Source: CAD feature listing. Evaluate the final solid. Frame: model axes, mm. Coordinates: 2 decimals unless noted, no trailing zeros. Loops run counter-clockwise (first coordinate to the right, second up) from the corner with the lowest first, then second, coordinate; pieces in that order, holes last. Notation, with made-up numbers: (52.5, 27.5) - (62.5, 27.5) arc R14 cw to (62.5, 40.5) - close; hole circle Ø6 at (64, 11.5). An arc over 180 degrees is marked (long way). Use one line per item in the form item = value. Start each with the question number.
Solid Edge part; units mm, degrees
sketch "Sketch1" plane through (0, 0, 0) normal (0, 0, 1) x (1, 0, 0)
  arc A0 (0, 6.3) -> (0.3, 6) centre (0.3, 6.3) ccw
  line L0 (0.3, 6) -> (7.7, 6)
  arc A1 (7.7, 6) -> (8, 6.3) centre (7.7, 6.3) ccw
  line L1 (8, 6.3) -> (8, 8.4)
  arc A2 (8, 8.4) -> (7.9, 8.5) centre (7.9, 8.4) ccw
  line L2 (7.9, 8.5) -> (5.8491, 8.5)
  arc A3 (5.8491, 8.5) -> (2.1509, 8.5) centre (4, 10) cw
  line L3 (2.1509, 8.5) -> (0.1, 8.5)
  arc A4 (0.1, 8.5) -> (0, 8.4) centre (0.1, 8.4) ccw
  line L4 (0, 8.4) -> (0, 6.3)
revolve "RevolvedProtrusion1" add sketch "Sketch1" angle 360 about axis through (100, 0, 0) along (-1, 0, 0)
properties part number "SKF_6001_ir"
(1) Mould query, pull axis Z, two halves, no side actions, for faces 1 (the face through (1.11, -1.84, 8.3)), 2 (the face through (8, 3, -6)), 3 (the face through (4, -6, 0)). Classes: +Z half, -Z half, draft (parallel to the pull), parting line (faces both ways), or undercut.
(2) Contact query for flat-ended pins moving along their axis: pin 1 (1 mm diameter, centred on x = 2.5, y = -6.5, fed in from +Z); pin 2 (2 mm diameter, centred on x = 1, y = -3.5, fed in from -Z); pin 3 (2 mm diameter, centred on x = 6, z = 5.5, fed in from +Y). Output: stop coordinate, or through.
(3) Cut plane A-A, the plane y = 0. Output: boundary loops of the cut face in (x, z).
(4) Cut plane D-D, the plane x = 3.75. Output: boundary loops of the cut face in (y, z), plus the area to 3 significant figures.
(5) Cut plane C-C, the plane x = 5.25. Output: boundary loops of the cut face in (y, z), plus the area to 3 significant figures.
(6) Material intervals for line 1 (Z direction, x = 6.5, y = 0); line 2 (Y direction, x = 1, z = -1.5), sorted ascending.
Recorded:
q1.face_1 = parting line
q1.face_2 = draft
q1.face_3 = undercut
q2.pin_1 = 5.88
q2.pin_2 = -8.12
q2.pin_3 = 7.21
q3.outline = (0, -8.4) arc R0.1 ccw to (0.1, -8.5) - (2.15, -8.5) arc R2.38 cw to (5.85, -8.5) - (7.9, -8.5) arc R0.1 ccw to (8, -8.4) - (8, -6.3) arc R0.3 ccw to (7.7, -6) - (0.3, -6) arc R0.3 ccw to (0, -6.3) - close; (0, 6.3) arc R0.3 ccw to (0.3, 6) - (7.7, 6) arc R0.3 ccw to (8, 6.3) - (8, 8.4) arc R0.1 ccw to (7.9, 8.5) - (5.85, 8.5) arc R2.38 cw to (2.15, 8.5) - (0.1, 8.5) arc R0.1 ccw to (0, 8.4) - close
q4.outline = circle Ø15.26 at (0, 0); hole circle Ø12 at (0, 0)
q4.area = 69.9 mm²
q5.outline = circle Ø15.95 at (0, 0); hole circle Ø12 at (0, 0)
q5.area = 86.6 mm²
q6.line_1 = -8.5 to -6, 6 to 8.5
q6.line_2 = -8.37 to -5.81, 5.81 to 8.37
